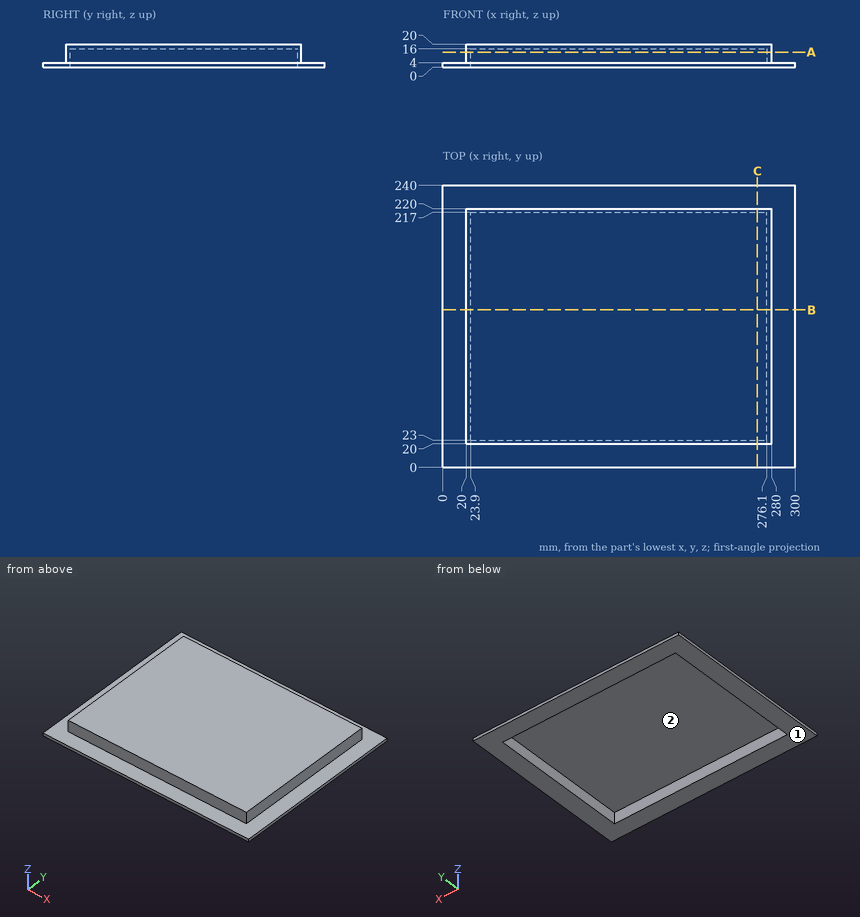
For this review, use the dimensioned drawing (mm, ordinates from the lowest corner) and the shaded views. Give positions to 0.01 mm unless a question says otherwise; leave off trailing zeros. Order: outer loops, then holes, each group sorted by start corner. A loop starts at its lowest first (then second) coordinate and runs counter-clockwise, first axis right, second up.
1) The part is to be moulded in two halves that separate along Y. For the marked faces 1 and 2, say which applies: released by +Y, released by -Y, zero draft, split by the parting line, or undercut.
2) Take a section at B-B (y = 134). Give the boundary of the cut face in (x, z).
3) Insertion check: pin 1 (4 mm diameter, centred on x = 141, z = 17.5, fed in from +Y); pin 2 (8 mm diameter, centred on x = 182, z = 14.5, fed in from -Y); pin 3 (8 mm diameter, centred on x = 172.5, y = 48, fed in from -Z). Each pin has a flat end and moves straight along its axis. Give the tip position at first contact, or say it passes through.
4) Wall thickness on line 1 (X direction, y = 166, z = 7.75); line 2 (X direction, y = 40.5, z = 2); line 3 (Y direction, x = 105, z = 4.25): over which ranges is each line inside the solid? List them lowest first.
5) Take a section at A-A (z = 13). Give the boundary of the cut face in (x, y).
6) Take a section at C-C (x = 268). Give the boundary of the cut face in (y, z).
Derived:
1. face 1: zero draft
1. face 2: undercut
2. outline: (0, 0) - (23.9, 0) - (23.9, 16) - (276.1, 16) - (276.1, 0) - (300, 0) - (300, 4) - (280, 4) - (280, 20) - (20, 20) - (20, 4) - (0, 4) - close
3. pin 1: stops at y = 220
3. pin 2: stops at y = 20
3. pin 3: stops at z = 16
4. line 1: x = 20 to 23.9, 276.1 to 280
4. line 2: x = 0 to 23.9, 276.1 to 300
4. line 3: y = 20 to 23, 217 to 220
5. outline: (20, 20) - (280, 20) - (280, 220) - (20, 220) - close; hole (23.9, 23) - (276.1, 23) - (276.1, 217) - (23.9, 217) - close
6. outline: (0, 0) - (23, 0) - (23, 16) - (217, 16) - (217, 0) - (240, 0) - (240, 4) - (220, 4) - (220, 20) - (20, 20) - (20, 4) - (0, 4) - close
